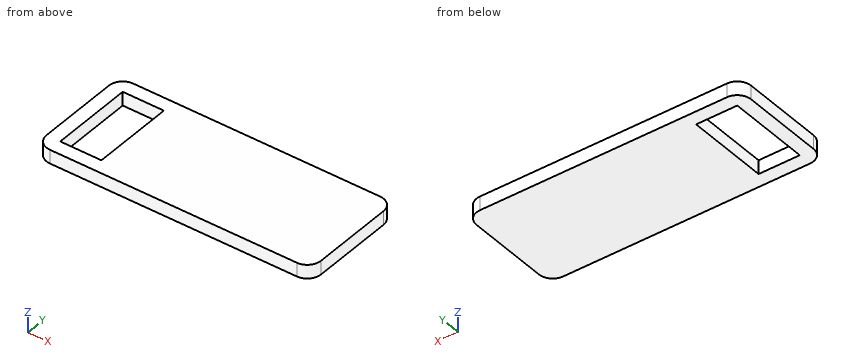
```python
from build123d import *

# Parameters (mm, degrees)
F0_W     = 100
F0_H     = 40
F0_W_2   = 15
F0_H_2   = 30
F1_DEPTH = 5
F2_R     = 5


with BuildPart() as f1:
    # F0 (on Top) → F1 (new body)
    with BuildSketch(Plane.XY):
        Rectangle(F0_W, F0_H)
        with Locations((-37.5, 0)):
            Rectangle(F0_W_2, F0_H_2, mode=Mode.SUBTRACT)
    extrude(amount=F1_DEPTH)

    # F2
    f2_edges = [f1.edges().sort_by_distance(p)[0] for p in [
        (-50, -20, 2.5),
        (50, -20, 2.5),
        (50, 20, 2.5),
        (-50, 20, 2.5),
    ]]
    fillet(f2_edges, radius=F2_R)


solid = f1.part
```
Design review of the part built by this model. Coordinates are the model's own, in mm. Coordinates: 2 decimals unless noted, no trailing zeros. Write each loop counter-clockwise with the first axis right and the second up, starting at its lowest first coordinate (ties: lowest second). Pieces come first, ordered by that corner, then holes.
1) Add section A-A (y = 1). Write out the cut boundary in (x, z), plus the area to 3 significant figures.
2) To check wall thickness, follow L1, parallel to X at y = 6.5, z = 2.2; L2, parallel to Y at x = -34.5, z = 1.6; L3, parallel to X at y = 18, z = 1.5. State the ranges of each line that lie inside material, in increasing order.
3) Add section C-C (x = -39.5). Write out the cut boundary in (y, z), plus the area to 3 significant figures.
4) Add section B-B (z = 0.85). Write out the cut boundary in (x, y), plus the area to 3 significant figures.
Check result:
1. outline: (-50, 0) - (-45, 0) - (-45, 5) - (-50, 5) - close; (-30, 0) - (50, 0) - (50, 5) - (-30, 5) - close
1. area: 425 mm2
2. L1: x = -50 to -45, -30 to 50
2. L2: y = -20 to -15, 15 to 20
2. L3: x = -49 to 49
3. outline: (-20, 0) - (-15, 0) - (-15, 5) - (-20, 5) - close; (15, 0) - (20, 0) - (20, 5) - (15, 5) - close
3. area: 50.0 mm2
4. outline: (-50, -15) arc R5 ccw to (-45, -20) - (45, -20) arc R5 ccw to (50, -15) - (50, 15) arc R5 ccw to (45, 20) - (-45, 20) arc R5 ccw to (-50, 15) - close; hole (-45, -15) - (-30, -15) - (-30, 15) - (-45, 15) - close
4. area: 3,530 mm2
